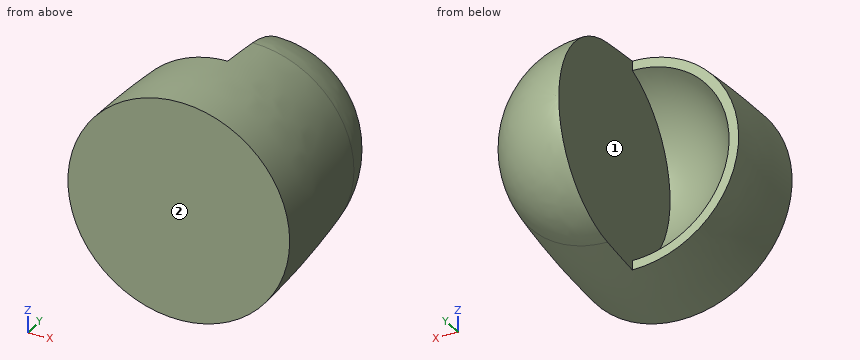
Autodesk Inventor part; units mm, degrees
ref_plane "YZ Plane" through (0, 0, 0) normal (1, 0, 0) x (0, 1, 0)
ref_plane "XZ Plane" through (0, 0, 0) normal (0, 1, 0) x (-1, 0, 0)
ref_plane "XY Plane" through (0, 0, 0) normal (0, 0, 1) x (1, 0, 0)
sketch "Эскиз1" plane through (0, 0, 0) normal (0, 0, 1) x (1, 0, 0)
  arc A0 (49.6078, 6.25) -> (0, 50) centre (0, 0) ccw
  line L0 (0, 0) -> (0, -250)
  circle A1 centre (0, -250) radius 25
  arc A2 (23.7255, -257.8804) -> (54.25, -60) centre (-545.6862, -68.75) ccw construction
  line L1 (54.25, -60) -> (0, -60)
  arc A3 (0, -50) -> (49.6078, 6.25) centre (0, 0) ccw construction
  line L2 (0, 0) -> (0, 50)
  arc A4 (0, 50) -> (0, -50) centre (0, 0) ccw construction
  arc A5 (54.25, -60) -> (49.6078, 6.25) centre (-545.6862, -68.75) ccw
  dimension "d2" = 50
  dimension "d0" = 100
  dimension "d1" = 250
  dimension "d3" = 600
  dimension "d4" = 60
revolve "Вращение1" add sketch "Эскиз1" angle 360 about axis through (0, 0, 0) along (0, -1, 0) contours A5 L1 L0 L2 A0
sketch "Эскиз2" plane through (0, 0, 0) normal (1, 0, 0) x (0, 1, 0)
  line L0 (6.25, 49.6078) -> (6.25, -49.6078) construction
  arc A0 (0, -50) -> (0, 50) centre (0, 0) ccw construction
  line L1 (0, -50) -> (0, 50)
  arc A1 (0, 50) -> (0, -50) centre (0, 0) ccw
  dimension "d6" = 100
revolve "Вращение2" cut sketch "Эскиз2" angle 180 about axis through (0, 0, -50) along (0, 0, -1)
sketch "Эскиз3" plane through (0, 0, 0) normal (0, 0, 1) x (1, 0, 0)
  line L0 (0, 6.25) -> (0, 50)
  arc A0 (-49.6078, 6.25) -> (-54.25, -60) centre (545.6862, -68.75) ccw
  line L1 (0, 50) -> (-52, 50)
  line L2 (-52, 50) -> (-52, -16.1078)
  line L3 (-52, -16.1078) -> (0, -16.1078)
  line L4 (0, -16.1078) -> (0, 50)
  point P0 (0, 0)
  dimension "d11" = 52
extrude "Выдавливание1" cut sketch "Эскиз3" along normal through all both and the other way through all
properties part number "ч ASY human dummy 01"
Part model, mm, in its own coordinate system. Face numbers are marked on the shaded views. Give positions to 0.01 mm unless a question says otherwise; leave off trailing zeros. Return JSON: item names as keys, results as strings.
1) Drill centre lines: line 1 (Y direction, x = -21, z = 45); line 2 (X direction, y = -32, z = 29); line 3 (X direction, y = -24.5, z = 39). Where is each one in solid material? Low to high.
Calculated:
{"line 1": "y = -60 to -16.11", "line 2": "x = -44.59 to -25.2, 0 to 44.59", "line 3": "x = -35.41 to -19.46, 0 to 35.41"}
2) Pull direction X, two halves, no side cores. Call the marked faces 1 and 2: released by +X, released by -X, zero draft, split by the parting line, or undercut.
Calculated:
{"face 1": "undercut", "face 2": "zero draft"}
3) Flat gauge pins, fed straight in: pin 1 Ø1 at (x, y) = (41, 4.5) entering from +Z; pin 2 Ø2 at (y, z) = (-33, 21) entering from -X; pin 3 Ø2 at (y, z) = (-25, -32) entering from -X. Where does each tip first touch, or does it go through?
Calculated:
{"pin 1": "stops at z = 29.03", "pin 2": "stops at x = -49.35", "pin 3": "stops at x = -42.64"}
